Solid Edge part; units mm, degrees
sketch "Sketch1" plane through (0, 0, 0) normal (0, 0, 1) x (1, 0, 0)
  line L0 (-0.0166, 6) -> (19.9834, 6)
  arc A0 (19.9834, 6) -> (19.9834, -6) centre (19.9834, 0) cw
  line L1 (19.9834, -6) -> (-0.0166, -6)
  arc A1 (-0.0166, -6) -> (-0.0166, 6) centre (-0.0166, 0) cw
extrude "Protrusion1" add sketch "Sketch1" along normal blind 4
hole "Hole_1" at (0, 0, 4) direction (0, 0, -1) diameter 5.2 end up to next
hole "Hole1" at (19.9834, 0, 4) direction (0, 0, -1) diameter 5.2 end up to next
properties material "Aluminum, 6061-T6"
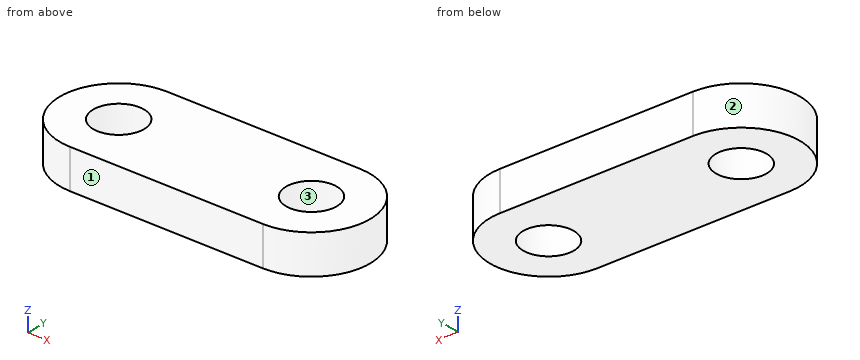
Geometry: final body of the model. Coordinates: model frame, mm. Face numbers are marked on the shaded views. Give positions to 0.01 mm unless a question says otherwise; leave off trailing zeros. Write each loop counter-clockwise with the first axis right and the second up, starting at its lowest first coordinate (ties: lowest second). Pieces come first, ordered by that corner, then holes. Notation, with made-up numbers: (60, 52) - (73, 52) arc R19 cw to (73, 87) - close; hole circle Ø4 at (1.5, 59.5). An arc over 180 degrees is marked (long way). Return JSON: item names as keys, results as strings. Group by question number.
1) First-contact query: P1, Ø2, axis at y = 4.5, z = 3.5, coming from the +X side. Flat tip, straight axial feed; report the tip coordinate or a pass-through.
2) Section B-B on x = 21. Return the cut outline in (y, z), plus the area to 3 significant figures.
3) Section A-A on y = 0. Return the cut outline in (x, z).
4) Line query: line 1 (X direction, y = 0, z = 1.1); line 2 (Y direction, x = 0, z = 1); line 3 (X direction, y = -0.75, z = 3.4). Output: solid intervals per line, ascending.
5) Mould query, pull axis Y, two halves, no side actions, for the marked faces 1, 2 and 3. Classes: released by +Y, released by -Y, zero draft, split by the parting line, or undercut.
6) Section C-C on z = 1.35. Return the cut outline in (x, y).
7) Section D-D on y = 1.5. Return the cut outline in (x, z), plus the area to 3 significant figures.
Filled in:
{
 "1": {"P1": "stops at x = 24.86"},
 "2": {"outline": "(-5.91, 0) - (-2.39, 0) - (-2.39, 4) - (-5.91, 4) - close; (2.39, 0) - (5.91, 0) - (5.91, 4) - (2.39, 4) - close", "area": "28.2 mm^2"},
 "3": {"outline": "(-6.02, 0) - (-2.6, 0) - (-2.6, 4) - (-6.02, 4) - close; (2.6, 0) - (17.38, 0) - (17.38, 4) - (2.6, 4) - close; (22.58, 0) - (25.98, 0) - (25.98, 4) - (22.58, 4) - close"},
 "4": {"line 1": "x = -6.02 to -2.6, 2.6 to 17.38, 22.58 to 25.98", "line 2": "y = -6 to -2.6, 2.6 to 6", "line 3": "x = -5.97 to -2.49, 2.49 to 17.49, 22.47 to 25.94"},
 "5": {"face 1": "released by -Y", "face 2": "split by the parting line", "face 3": "undercut"},
 "6": {"outline": "(-0.02, -6) - (19.98, -6) arc R6 ccw to (19.98, 6) - (-0.02, 6) arc R6 ccw to start; hole circle Ø5.2 at (0, 0); hole circle Ø5.2 at (19.98, 0)"},
 "7": {"outline": "(-5.83, 0) - (-2.12, 0) - (-2.12, 4) - (-5.83, 4) - close; (2.12, 0) - (17.86, 0) - (17.86, 4) - (2.12, 4) - close; (22.11, 0) - (25.79, 0) - (25.79, 4) - (22.11, 4) - close", "area": "92.5 mm^2"}
}
